from build123d import *

# Parameters (mm, degrees)
EXTRUDE1_DEPTH     = 26
SKETCH24_W         = 77.68
SKETCH24_H         = 32
CUT_EXTRUDE1_DEPTH = 89.181885328
FILLET1_R          = 6.35
SKETCH25_W         = 0.75
SKETCH25_H         = 12.75
CUT_EXTRUDE2_DEPTH = 100.95771556
CUT_EXTRUDE5_DEPTH = 85.627093179


with BuildPart() as part:
    # Sketch1 → Extrude1 (new, symmetric)
    with BuildSketch(Plane.XY):
        Polygon((0, 0), (0, 21.25), (5, 21.25), (5, 5), (82.68, 5), (82.68, 0), align=None)
    extrude(amount=EXTRUDE1_DEPTH, both=True)

    # Sketch24 → Cut-Extrude1 (cut, through all)
    with BuildSketch(Plane(origin=(0, 5, 0), x_dir=(1, 0, 0), z_dir=(0, 1, 0))):
        with Locations((43.84, 10)):
            Rectangle(SKETCH24_W, SKETCH24_H)
    extrude(amount=-CUT_EXTRUDE1_DEPTH, mode=Mode.SUBTRACT)

    # Fillet1
    fillet1_edges = [part.edges().sort_by_distance(p)[0] for p in [
        (5, 2.5, 6),
    ]]
    fillet(fillet1_edges, radius=FILLET1_R)

    # Sketch25 → Cut-Extrude2 (cut, through all)
    with BuildSketch(Plane.XY.offset(26)):
        with Locations((0.375, 6.375)):
            Rectangle(SKETCH25_W, SKETCH25_H)
    extrude(amount=-CUT_EXTRUDE2_DEPTH, mode=Mode.SUBTRACT)

    # Sketch30 → Cut-Extrude5 (cut, through all)
    with BuildSketch(Plane(origin=(5, 0, 0), x_dir=(0, 0, -1), z_dir=(1, 0, 0))):
        with BuildLine():
            Line((26, 0), (5, 0))
            Line((5, 0), (5, 10.075))
            ThreePointArc((5, 10.075), (5.92993597, 12.32006403), (8.175, 13.25))
            Line((8.175, 13.25), (26, 13.25))
            Line((26, 13.25), (26, 0))
        make_face()
    extrude(amount=-CUT_EXTRUDE5_DEPTH, mode=Mode.SUBTRACT)


solid = part.part
For this review, take the finished solid that the model builds, in its own axes (mm). A direction names the side the tool comes from. Give positions to 0.01 mm unless a question says otherwise; leave off trailing zeros. Loops run counter-clockwise (first coordinate to the right, second up) from the corner with the lowest first, then second, coordinate; pieces in that order, holes last.
Item 1: Take a section at B-B, the plane y = 1.5. State the section outline as (x, z) points.
Item 2: For line 1 along X through (y, z) = (13.5, 22); line 2 along Z through (x, y) = (38, 2.5), list the stretches that pass through material, from the lowest coordinate up.
Item 3: Take a section at A-A, the plane z = 15. State the section outline as (x, y) points, and give its area (3 significant figures).
Item 4: Tool access review of faces 1 (the flat face through (43, 5, 16)), 2 (the flat face through (42, 0, 14)), 3 (the flat face through (3, 13.25, -17)), 4 (the flat face through (0.75, 6, 10)), 5 (the flat face through (47, 3, 6)): name each direction out of +Z, -Z, +X, -X, +Y, -Y from which nothing blocks a thin tool from reaching the whole face with its end or side.
Item 5: Insertion check: pin 1 (4 mm diameter, centred on x = 25.5, z = 7.5, fed in from +Y); pin 2 (2 mm diameter, centred on x = 2.5, y = 6, fed in from -Z); pin 3 (8 mm diameter, centred on y = 3, z = 17.5, fed in from -X); pin 4 (2 mm diameter, centred on y = 10.5, z = -17.5, fed in from -X). Each pin has a flat end and moves straight along its axis. Give the tip position at first contact, or say it passes through.
Item 6: Take a section at D-D, the plane z = -4. State the section outline as (x, y) points.
Item 7: Take a section at C-C, the plane x = 22.5. State the section outline as (y, z) points.
Calculated:
1. outline: (0.75, -5) - (5, -5) - (5, -0.35) arc R6.35 cw to (11.35, 6) - (82.68, 6) - (82.68, 26) - (0.75, 26) - close
2. line 1: x = 0 to 5
2. line 2: z = 6 to 26
3. outline: (0, 12.75) - (0.75, 12.75) - (0.75, 0) - (82.68, 0) - (82.68, 5) - (5, 5) - (5, 21.25) - (0, 21.25) - close
3. area: 485 mm2
4. face 1: +Z, -Z, +X, +Y
4. face 2: +Z, -Z, +X, -X, -Y
4. face 3: -Z, +X, -X, -Y
4. face 4: +Z, -Z, -X, -Y
4. face 5: -Z, +X, +Y, -Y
5. pin 1: stops at y = 5
5. pin 2: stops at z = -5
5. pin 3: stops at x = 0.75
5. pin 4: passes through
6. outline: (0, 12.75) - (0.75, 12.75) - (0.75, 0) - (5, 0) - (5, 21.25) - (0, 21.25) - close
7. outline: (0, 6) - (5, 6) - (5, 26) - (0, 26) - close
